Geometry check sheet. Reference: the model listing, model coordinates, mm. Face numbers are marked on the shaded views. A direction names the side the tool comes from. Coordinates: 2 decimals unless noted, no trailing zeros. Write each loop counter-clockwise with the first axis right and the second up, starting at its lowest first coordinate (ties: lowest second). Pieces come first, ordered by that corner, then holes. Notation, with made-up numbers: (44.5, -25.5) - (102.5, -25.5) arc R11 cw to (102.5, -11.5) - close; hole circle Ø6 at (81, 55.25). An arc over 180 degrees is marked (long way). Answer as a JSON object with one key per item and string values. Group by question number.
from build123d import *

# Parameters (mm, degrees)
F0_R            = 12.5
F1_DEPTH        = 122.5
F2_R            = 12.5
F3_DEPTH        = 65
F4_DEPTH        = 23
F5_DEPTH        = 25
F6_R            = 19
F7_DEPTH        = 3
F8_R            = 5.5
F9_DEPTH        = 28
F11_D           = 5.5
F11_DEPTH       = 100
F11_CSINK_D     = 11
F11_CSINK_ANGLE = 90


with BuildPart() as f1:
    # F0 (on Top) → F1 (new body)
    with BuildSketch(Plane.XY):
        Circle(F0_R)
    extrude(amount=F1_DEPTH)

    # F2 (on Right) → F3 (join)
    with BuildSketch(Plane.YZ):
        Circle(F2_R)
    extrude(amount=F3_DEPTH)

    # F2 (on Right) → F4 (join)
    with BuildSketch(Plane.YZ):
        Circle(F2_R)
    extrude(amount=-F4_DEPTH)

    # F0 (on Top) → F5 (join)
    with BuildSketch(Plane.XY):
        Circle(F0_R)
    extrude(amount=-F5_DEPTH)

    # F6 (on face) → F7 (join)
    with BuildSketch(Plane.XY.offset(122.5)):
        Circle(F6_R)
    extrude(amount=F7_DEPTH)

    # F8 (on face) → F9 (cut)
    with BuildSketch(Plane(origin=(-23, 0, 0), x_dir=(0, -1, 0), z_dir=(-1, 0, 0))):
        Circle(F8_R)
    extrude(amount=-F9_DEPTH, mode=Mode.SUBTRACT)

    # F11
    with Locations(Plane(origin=(5, 0, 0), x_dir=(0, -1, 0), z_dir=(-1, 0, 0))):
        with Locations((0, 0)):
            CounterSinkHole(F11_D / 2, F11_CSINK_D / 2, depth=F11_DEPTH, counter_sink_angle=F11_CSINK_ANGLE)


solid = f1.part
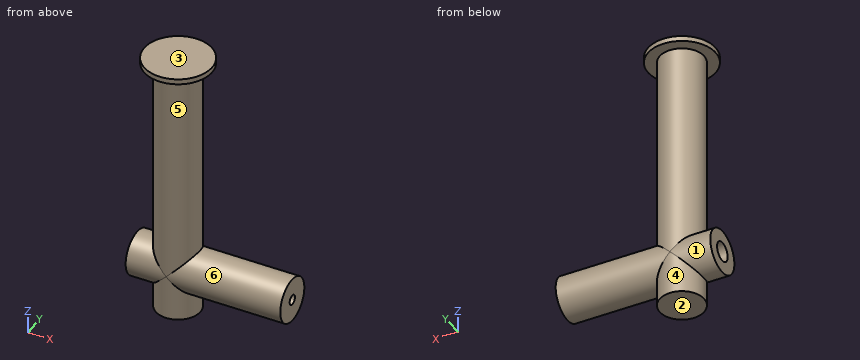
(1) Set-up check for the marked faces 4, 5 and 6: record each of +Z, -Z, +X, -X, +Y, -Y from which the full face is reachable in a straight line by a thin tool's end or side.
(2) Draft check along Z on the marked faces 1, 2 and 3. Enter one of: +Z half, -Z half, draft (parallel to the pull), parting line (faces both ways), or undercut.
(3) Section check D-D (x = -10). Record the cut outline in (y, z).
(4) Section check C-C (z = 38.5). Record the cut outline in (x, y).
(5) Section check A-A (y = 0). Record the cut outline in (x, z).
(6) Material ranges on L1, parallel to Z at x = -9.25, y = 0; L2, parallel to Z at x = 38, y = 0; L3, parallel to X at y = 0, z = 119, recorded low to high. Write a range as [from, to].
(7) Section check B-B (x = 2). Record the cut outline in (y, z).
(8) Gauge pin test, flat ends, axial feed: pin 1 (3 mm diameter, centred on x = 37, y = 12, fed in from +Z); pin 2 (10 mm diameter, centred on y = 0, z = 0, fed in from -X); pin 3 (5 mm diameter, centred on x = -13.5, z = 33, fed in from -Y). Record the tip position at first contact, or that the pin passes through.
Conclusion:
{
 "1": {"face 4": "-Z", "face 5": "none", "face 6": "+X"},
 "2": {"face 1": "undercut", "face 2": "-Z half", "face 3": "+Z half"},
 "3": {"outline": "(-16.16, 122.5) - (-7.5, 122.5) - (-7.5, 10) arc R12.5 ccw to (-7.5, -10) - (-7.5, -25) - (7.5, -25) - (7.5, -10) arc R12.5 ccw to (7.5, 10) - (7.5, 122.5) - (16.16, 122.5) - (16.16, 125.5) - (-16.16, 125.5) - close; hole circle Ø11 at (0, 0)"},
 "4": {"outline": "circle Ø25 at (0, 0)"},
 "5": {"outline": "(-23, -12.5) - (-12.5, -12.5) - (-12.5, -25) - (12.5, -25) - (12.5, -12.5) - (65, -12.5) - (65, -2.75) - (7.75, -2.75) - (5, -5.5) - (-23, -5.5) - close; (-23, 5.5) - (5, 5.5) - (7.75, 2.75) - (65, 2.75) - (65, 12.5) - (12.5, 12.5) - (12.5, 122.5) - (19, 122.5) - (19, 125.5) - (-19, 125.5) - (-19, 122.5) - (-12.5, 122.5) - (-12.5, 12.5) - (-23, 12.5) - close"},
 "6": {"L1": "z = [-25, -5.5], [5.5, 125.5]", "L2": "z = [-12.5, -2.75], [2.75, 12.5]", "L3": "x = [-12.5, 12.5]"},
 "7": {"outline": "(-18.89, 122.5) - (-12.34, 122.5) - (-12.34, 2) arc R12.5 ccw to (-12.34, -2) - (-12.34, -25) - (12.34, -25) - (12.34, -2) arc R12.5 ccw to (12.34, 2) - (12.34, 122.5) - (18.89, 122.5) - (18.89, 125.5) - (-18.89, 125.5) - close; hole circle Ø11 at (0, 0)"},
 "8": {"pin 1": "stops at z = 6.78", "pin 2": "stops at x = 5.5", "pin 3": "stops at y = -5.94"}
}
